Input: part model. Units: mm. Frame: model coordinates. Face numbers are marked on the shaded views. A direction names the side the tool comes from. Round coordinates to 2 decimals unless told otherwise and drop trailing zeros. Loops run counter-clockwise (first coordinate to the right, second up) from the corner with the lowest first, then second, coordinate; pieces in that order, holes last.
(1) Cut plane C-C, the plane x = -69. Output: boundary loops of the cut face in (y, z), and give its area (3 significant figures).
(2) First-contact query: pin 1 Ø5 at (x, y) = (-4, 39) entering from -Z; pin 2 Ø1.5 at (y, z) = (23, 7) entering from +X; pin 3 Ø3 at (x, y) = (-4, 39) entering from +Z; pin 4 Ø5 at (x, y) = (-6.5, 22) entering from -Z. Flat tips, straight axial feed; report the tip coordinate or a pass-through.
(3) Draft query along X for the marked faces 4, 5 and 6. Return one class per face: released by +X, released by -X, zero draft, split by the parting line, or undercut.
(4) Access query for the marked faces 1, 2 and 3. Directions: +Z, -Z, +X, -X, +Y, -Y. A direction counts if a zero-diameter tool reaches every point of the face in a straight line with its end or side. Return the directions, or none.
(5) Cut plane D-D, the plane y = 13.5. Output: boundary loops of the cut face in (x, z).
(6) Cut plane A-A, the plane x = -35. Output: boundary loops of the cut face in (y, z), and give its area (3 significant figures).
(7) Cut plane B-B, the plane z = 3. Output: boundary loops of the cut face in (x, y).
(8) Line query: line 1 (X direction, y = 4, z = 4.25); line 2 (X direction, y = 4, z = 0.95); line 3 (X direction, y = 39, z = 1.05). Output: solid intervals per line, ascending.
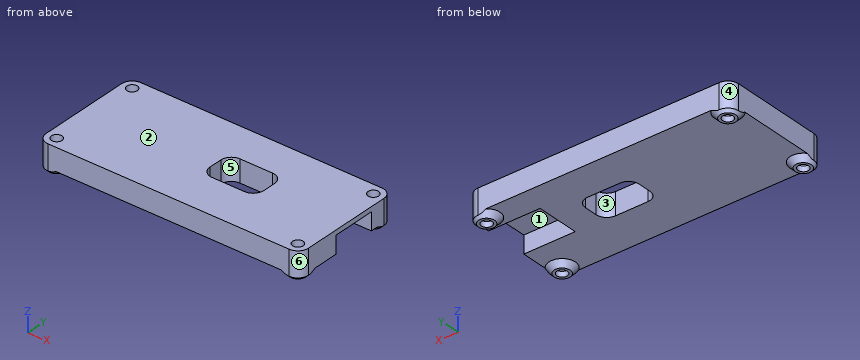
from build123d import *

# Parameters (mm, degrees)
SKETCH3_W           = 99
SKETCH3_H           = 43
SKETCH3_R           = 2
BOSS_EXTRUDE2_DEPTH = 8.399995141
BOSS_EXTRUDE3_START = 2
SKETCH4_R           = 3
SKETCH4_R_2         = 2
BOSS_EXTRUDE3_DEPTH = 2
CHAMFER1_SIZE       = 2
SKETCH5_W           = 8.599999433
SKETCH5_H           = 16.3
CUT_EXTRUDE1_DEPTH  = 19.390997243
CUT_EXTRUDE2_REACH  = 110.262
SKETCH6_W           = 20.299990895
SKETCH6_H           = 13.000003078
FILLET1_R           = 4


# Some blends are built 0.0001 mm under size
with BuildPart() as part:
    # Sketch3 → Boss-Extrude2 (new body)
    with BuildSketch(Plane.XY.offset(2)):
        with Locations((-49.5, 21.5)):
            Rectangle(SKETCH3_W, SKETCH3_H)
        with Locations(Location((-95, 39, 0), (0, 0, 270))):
            Circle(SKETCH3_R, mode=Mode.SUBTRACT)
        with Locations(Location((-95, 4, 0), (0, 0, 270))):
            Circle(SKETCH3_R, mode=Mode.SUBTRACT)
        with Locations(Location((-4, 4, 0), (0, 0, 270))):
            Circle(SKETCH3_R, mode=Mode.SUBTRACT)
        with Locations(Location((-4, 39, 0), (0, 0, 270))):
            Circle(SKETCH3_R, mode=Mode.SUBTRACT)
    extrude(amount=BOSS_EXTRUDE2_DEPTH)

    # Sketch4 → Boss-Extrude3 (add)
    # profile 1 of 4: a face of its own
    with BuildSketch(Plane(origin=(0, 0, 2), x_dir=(-1, 0, 0), z_dir=(0, 0, -1)).offset(BOSS_EXTRUDE3_START)):
        with Locations(Location((4, 39, 0), (0, 0, 180))):
            Circle(SKETCH4_R)
        with Locations(Location((4, 39, 0), (0, 0, 270))):
            Circle(SKETCH4_R_2, mode=Mode.SUBTRACT)
    # profile 2 of 4: a face of its own
    with BuildSketch(Plane(origin=(0, 0, 2), x_dir=(-1, 0, 0), z_dir=(0, 0, -1)).offset(BOSS_EXTRUDE3_START)):
        with Locations(Location((95, 39, 0), (0, 0, 180))):
            Circle(SKETCH4_R)
        with Locations(Location((95, 39, 0), (0, 0, 270))):
            Circle(SKETCH4_R_2, mode=Mode.SUBTRACT)
    # profile 3 of 4: a face of its own
    with BuildSketch(Plane(origin=(0, 0, 2), x_dir=(-1, 0, 0), z_dir=(0, 0, -1)).offset(BOSS_EXTRUDE3_START)):
        with Locations(Location((95, 4, 0), (0, 0, 180))):
            Circle(SKETCH4_R)
        with Locations(Location((95, 4, 0), (0, 0, 270))):
            Circle(SKETCH4_R_2, mode=Mode.SUBTRACT)
    # profile 4 of 4: a face of its own
    with BuildSketch(Plane(origin=(0, 0, 2), x_dir=(-1, 0, 0), z_dir=(0, 0, -1)).offset(BOSS_EXTRUDE3_START)):
        with Locations(Location((4, 4, 0), (0, 0, 180))):
            Circle(SKETCH4_R)
        with Locations(Location((4, 4, 0), (0, 0, 270))):
            Circle(SKETCH4_R_2, mode=Mode.SUBTRACT)
    extrude(amount=-BOSS_EXTRUDE3_DEPTH)

    # Chamfer1
    # the kernel refuses this chamfer: 2 mm, written as the material it adds along each edge
    with BuildSketch(Plane(origin=(-4, 39, 2), x_dir=(1, 0, 0), z_dir=(0, 1, 0))) as chamfer1_piece_1_section:
        Polygon((3 + CHAMFER1_SIZE, 0), (3, CHAMFER1_SIZE), (3, 0), align=None)
    chamfer1_piece_1 = revolve(axis=Axis((-4, 39, 2), (0, 0, -1)), mode=Mode.PRIVATE)
    chamfer1_piece_1 = split(chamfer1_piece_1, bisect_by=Plane(origin=(-8.002812408, 43, 1.053756135), z_dir=(0, -1, 0)), keep=Keep.TOP, mode=Mode.PRIVATE)
    chamfer1_piece_1 = split(chamfer1_piece_1, bisect_by=Plane(origin=(0, 39, 1.053756135), z_dir=(-1, 0, 0)), keep=Keep.TOP, mode=Mode.PRIVATE)
    chamfer1_piece_1 = split(chamfer1_piece_1, bisect_by=Plane(origin=(-8.002812408, 39, 0), z_dir=(0, 0, 1)), keep=Keep.TOP, mode=Mode.PRIVATE)
    add(chamfer1_piece_1)
    with BuildSketch(Plane(origin=(-95, 39, 2), x_dir=(1, 0, 0), z_dir=(0, 1, 0))) as chamfer1_piece_2_section:
        Polygon((3 + CHAMFER1_SIZE, 0), (3, CHAMFER1_SIZE), (3, 0), align=None)
    chamfer1_piece_2 = revolve(axis=Axis((-95, 39, 2), (0, 0, -1)), mode=Mode.PRIVATE)
    chamfer1_piece_2 = split(chamfer1_piece_2, bisect_by=Plane(origin=(-92.655832372, 43, 1.739278981), z_dir=(0, -1, 0)), keep=Keep.TOP, mode=Mode.PRIVATE)
    chamfer1_piece_2 = split(chamfer1_piece_2, bisect_by=Plane(origin=(-99, 34.939782567, 1.739278981), z_dir=(1, 0, 0)), keep=Keep.TOP, mode=Mode.PRIVATE)
    chamfer1_piece_2 = split(chamfer1_piece_2, bisect_by=Plane(origin=(-92.655832372, 34.939782567, 0), z_dir=(0, 0, 1)), keep=Keep.TOP, mode=Mode.PRIVATE)
    add(chamfer1_piece_2)
    with BuildSketch(Plane(origin=(-95, 4, 2), x_dir=(1, 0, 0), z_dir=(0, 1, 0))) as chamfer1_piece_3_section:
        Polygon((3 + CHAMFER1_SIZE, 0), (3, CHAMFER1_SIZE), (3, 0), align=None)
    chamfer1_piece_3 = revolve(axis=Axis((-95, 4, 2), (0, 0, -1)), mode=Mode.PRIVATE)
    chamfer1_piece_3 = split(chamfer1_piece_3, bisect_by=Plane(origin=(-99, 0.533462766, 1.053756132), z_dir=(1, 0, 0)), keep=Keep.TOP, mode=Mode.PRIVATE)
    chamfer1_piece_3 = split(chamfer1_piece_3, bisect_by=Plane(origin=(-92.998593795, 0, 1.053756132), z_dir=(0, 1, 0)), keep=Keep.TOP, mode=Mode.PRIVATE)
    chamfer1_piece_3 = split(chamfer1_piece_3, bisect_by=Plane(origin=(-92.998593795, 0.533462766, 0), z_dir=(0, 0, 1)), keep=Keep.TOP, mode=Mode.PRIVATE)
    add(chamfer1_piece_3)
    with BuildSketch(Plane(origin=(-4, 4, 2), x_dir=(1, 0, 0), z_dir=(0, 1, 0))) as chamfer1_piece_4_section:
        Polygon((3 + CHAMFER1_SIZE, 0), (3, CHAMFER1_SIZE), (3, 0), align=None)
    chamfer1_piece_4 = revolve(axis=Axis((-4, 4, 2), (0, 0, -1)), mode=Mode.PRIVATE)
    chamfer1_piece_4 = split(chamfer1_piece_4, bisect_by=Plane(origin=(0, 4, 1.053756135), z_dir=(-1, 0, 0)), keep=Keep.TOP, mode=Mode.PRIVATE)
    chamfer1_piece_4 = split(chamfer1_piece_4, bisect_by=Plane(origin=(-8.002812408, 0, 1.053756135), z_dir=(0, 1, 0)), keep=Keep.TOP, mode=Mode.PRIVATE)
    chamfer1_piece_4 = split(chamfer1_piece_4, bisect_by=Plane(origin=(-8.002812408, 4, 0), z_dir=(0, 0, 1)), keep=Keep.TOP, mode=Mode.PRIVATE)
    add(chamfer1_piece_4)

    # Sketch5 → Cut-Extrude1 (cut)
    with BuildSketch(Plane(origin=(0, 0, 0), x_dir=(0, 0, -1), z_dir=(1, 0, 0))):
        with Locations((-4.299999717, 25.013003939)):
            Rectangle(SKETCH5_W, SKETCH5_H)
    extrude(amount=-CUT_EXTRUDE1_DEPTH, mode=Mode.SUBTRACT)

    # Sketch6 → Cut-Extrude2 (cut, up to next)
    with BuildSketch(Plane(origin=(0, 0, 2), x_dir=(-1, 0, 0), z_dir=(0, 0, -1)), mode=Mode.PRIVATE) as cut_extrude2_sk1:
        with Locations((40.099996563, 22.600000838)):
            Rectangle(SKETCH6_W, SKETCH6_H)
    cut_extrude2_tool1 = extrude(cut_extrude2_sk1.sketch, amount=-CUT_EXTRUDE2_REACH, mode=Mode.PRIVATE) & part.part
    add(cut_extrude2_tool1.solids().sort_by_distance((-40.099997, 22.600001, 2))[0], mode=Mode.SUBTRACT)

    # Fillet1
    fillet1_edges = [part.edges().sort_by_distance(p)[0] for p in [
        (-50.249992011, 16.099999299, 6.19999757),
        (-50.249992011, 29.100002377, 6.19999757),
        (-29.950001116, 29.100002377, 6.19999757),
        (-29.950001116, 16.099999299, 6.19999757),
        (-99, 0, 6.19999757),
        (0, 0, 6.19999757),
        (0, 43, 6.19999757),
        (-99, 43, 6.19999757),
    ]]
    fillet(fillet1_edges, radius=FILLET1_R - 0.0001)  # a hair under: the kernel refuses the full size


solid = part.part
Reported:
1. outline: (0, 2) - (43, 2) - (43, 10.4) - (0, 10.4) - close
1. area: 361 mm2
2. pin 1: stops at z = 0
2. pin 2: stops at x = -19.39
2. pin 3: passes through
2. pin 4: stops at z = 8.6
3. face 4: released by -X
3. face 5: undercut
3. face 6: released by +X
4. face 1: -Z, +X
4. face 2: +Z, +X, -X, +Y, -Y
4. face 3: +Z, -Z
5. outline: (-99, 2) - (0, 2) - (0, 10.4) - (-99, 10.4) - close
6. outline: (0, 2) - (16.1, 2) - (16.1, 10.4) - (0, 10.4) - close; (29.1, 2) - (43, 2) - (43, 10.4) - (29.1, 10.4) - close
6. area: 252 mm2
7. outline: (-99, 4) arc R4 ccw to (-95, 0) - (-4, 0) arc R4 ccw to (0, 4) - (0, 16.86) - (-19.39, 16.86) - (-19.39, 33.16) - (0, 33.16) - (0, 39) arc R4 ccw to (-4, 43) - (-95, 43) arc R4 ccw to (-99, 39) - close; hole circle Ø4 at (-95, 4); hole circle Ø4 at (-95, 39); hole (-50.25, 20.1) arc R4 ccw to (-46.25, 16.1) - (-33.95, 16.1) arc R4 ccw to (-29.95, 20.1) - (-29.95, 25.1) arc R4 ccw to (-33.95, 29.1) - (-46.25, 29.1) arc R4 ccw to (-50.25, 25.1) - close; hole circle Ø4 at (-4, 4); hole circle Ø4 at (-4, 39)
8. line 1: x = -99 to -97, -93 to -6, -2 to 0
8. line 2: x = -98.95 to -97, -93 to -91.05, -7.95 to -6, -2 to -0.05
8. line 3: x = -99 to -97, -93 to -90.95, -8.05 to -6, -2 to 0
